```python
from build123d import *

# Parameters (mm, degrees)
SKETCH1_W           = 50
SKETCH1_H           = 41
BOSS_EXTRUDE1_DEPTH = 3
CUT_EXTRUDE1_DEPTH  = 47.19523785
FILLET1_R           = 2


with BuildPart() as part:
    # Sketch1 → Boss-Extrude1 (new body)
    with BuildSketch(Plane.XY):
        with Locations((-5, -14.5)):
            Rectangle(SKETCH1_W, SKETCH1_H)
    extrude(amount=BOSS_EXTRUDE1_DEPTH)

    # Sketch2 → Cut-Extrude1 (cut, through all)
    with BuildSketch(Plane.XY):
        with BuildLine():
            Line((-30, 0), (-0.5, 0))
            ThreePointArc((-0.5, 0), (0.353553391, 0.353553391), (0, -0.5))
            Line((0, -0.5), (0, -2.5))
            ThreePointArc((0, -2.5), (0.353553391, -3.353553391), (-0.5, -3))
            Line((-0.5, -3), (-30, -3))
            Line((-30, -3), (-30, 0))
        make_face()
    extrude(amount=CUT_EXTRUDE1_DEPTH, mode=Mode.SUBTRACT)

    # Fillet1
    fillet1_edges = [part.edges().sort_by_distance(p)[0] for p in [
        (-30, 0, 1.5),
        (-30, -3, 1.5),
    ]]
    fillet(fillet1_edges, radius=FILLET1_R)


solid = part.part
```
Could you check a few things on this model? Use its own coordinates, in mm. A direction names the side the tool comes from. Give positions to 0.01 mm unless a question says otherwise; leave off trailing zeros. Write each loop counter-clockwise with the first axis right and the second up, starting at its lowest first coordinate (ties: lowest second). Pieces come first, ordered by that corner, then holes. Notation, with made-up numbers: (-39, 41) - (-23, 41) arc R11 ccw to (-23, 62) - close; hole circle Ø3 at (-17.5, 13). An arc over 180 degrees is marked (long way). One line per item, written item: value. Start each with the question number.
Item 1: Which directions (+Z, -Z, +X, -X, +Y, -Y) give clear straight access to the entire face, cutting with the end or side of a thin tool? Please do faces 1 (the face through (-14, -3, 1)), 2 (the face through (0.4, -3.3, 1.5)).
Item 2: I'm going to push flat-ended pins straight in: pin 1 (1 mm diameter, centred on y = -2, z = 2, fed in from -X); pin 2 (0.9 mm diameter, centred on x = 0, y = 0, fed in from +Z). Where does each tip first touch, or does it pass through?
Item 3: Imagine slicing it at A-A, the plane x = -9.5. List the corners of the cut face in (y, z) for me.
Item 4: Imagine slicing it at B-B, the plane z = 1.65. List the corners of the cut face in (x, y) for me, and give its area (3 significant figures).
Item 5: Please list where these lines run through material, in increasing order: line 1 (Y direction, x = -21.5, z = 2.7); line 2 (X direction, y = 1, z = 2.6). Write a range as from..to.
Item 6: If we mould it in two halves opening along Y, with no side actions, what happens to faces 3 (the face through (-14, 0, 1)), 4 (the face through (-5, -35, 1)), 5 (the face through (-5, -14, 3))? For each: +Y half, -Y half, draft (parallel to the pull), parting line (faces both ways), or undercut.
Geometry says:
1. face 1: +Z, -Z, -X
1. face 2: +Z, -Z
2. pin 1: x = 0
2. pin 2: through
3. outline: (-35, 0) - (-3, 0) - (-3, 3) - (-35, 3) - close; (0, 0) - (6, 0) - (6, 3) - (0, 3) - close
4. outline: (-30, -35) - (20, -35) - (20, 6) - (-30, 6) - (-30, 2) arc R2 ccw to (-28, 0) - (-0.5, 0) arc R0.5 cw (long way) to (0, -0.5) - (0, -2.5) arc R0.5 cw (long way) to (-0.5, -3) - (-28, -3) arc R2 ccw to (-30, -5) - close
4. area: 1,960 mm^2
5. line 1: -35..-3, 0..6
5. line 2: -29.73..20
6. face 3: undercut
6. face 4: -Y half
6. face 5: draft
